Drawing for the job (mm, zero at the part's lowest x, y, z). Round coordinates to 2 decimals unless told otherwise and drop trailing zeros. Write each loop counter-clockwise with the first axis right and the second up, starting at its lowest first coordinate (ties: lowest second). Pieces come first, ordered by that corner, then holes. Notation, with made-up numbers: (-32, -35.5) - (13, -35.5) arc R19 cw to (13, -17.5) - close; hole circle Ø1 at (-30, 57.5). An arc over 180 degrees is marked (long way). Answer in a Markdown table with one row per item.
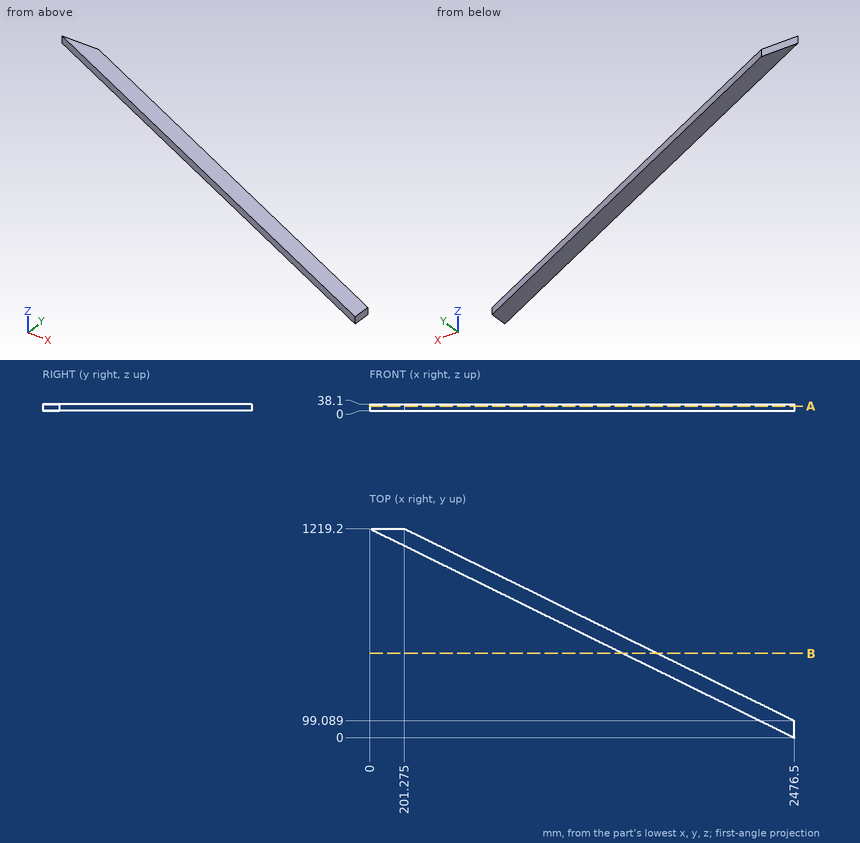
Q1. Drill centre lines: line 1 (Y direction, x = 1352.5, z = 9) (1 decimal); line 2 (Y direction, x = 1480.5, z = 23); line 3 (X direction, y = 882, z = 36) (1 decimal). Where is each one in solid material? Low to high.
Computed:
| item | result |
|---|---|
| line 1 | y = 553.4 to 652.4 |
| line 2 | y = 490.34 to 589.43 |
| line 3 | x = 684.9 to 886.2 |
Q2. Saw through at B-B on y = 491. List the corners of the cut face in (x, z), then the cut area to 3 significant figures.
Computed:
| item | result |
|---|---|
| outline | (1479.16, 0) - (1680.43, 0) - (1680.43, 38.1) - (1479.16, 38.1) - close |
| area | 7,670 mm2 |
Q3. Saw through at A-A on z = 25. List the corners of the cut face in (x, y) (1 decimal).
Computed:
| item | result |
|---|---|
| outline | (0, 1219.2) - (2476.5, 0) - (2476.5, 99.1) - (201.3, 1219.2) - close |
Q4. Flat gauge pins, fed straight in: pin 1 (12 mm diameter, centred on x = 1681.5, z = 4, fed in from -Y); pin 2 (4 mm diameter, centred on x = 1679, z = 29, fed in from +Y); pin 3 (5 mm diameter, centred on x = 292, z = 26, fed in from -Y) (1 decimal). Where does each tip first touch, or does it go through?
Computed:
| item | result |
|---|---|
| pin 1 | stops at y = 388.43 |
| pin 2 | stops at y = 492.69 |
| pin 3 | stops at y = 1074.2 |
